```python
from build123d import *

# Parameters (mm, degrees)
SKETCH1_W           = 48
SKETCH1_H           = 300
SKETCH1_R           = 7
SKETCH1_R_2         = 2
BOSS_EXTRUDE1_DEPTH = 5
CHAMFER1_SIZE       = 3
CUT_EXTRUDE1_DEPTH  = 304.856874202


with BuildPart() as part:
    # Sketch1 → Boss-Extrude1 (new body)
    with BuildSketch(Plane.XY):
        with Locations((24, -150)):
            Rectangle(SKETCH1_W, SKETCH1_H)
        with Locations((24, -160)):
            Circle(SKETCH1_R, mode=Mode.SUBTRACT)
        with Locations((8, -144)):
            Circle(SKETCH1_R_2, mode=Mode.SUBTRACT)
        with Locations((16, -144)):
            Circle(SKETCH1_R_2, mode=Mode.SUBTRACT)
        with Locations((24, -144)):
            Circle(SKETCH1_R_2, mode=Mode.SUBTRACT)
        with Locations((32, -144)):
            Circle(SKETCH1_R_2, mode=Mode.SUBTRACT)
        with Locations((40, -144)):
            Circle(SKETCH1_R_2, mode=Mode.SUBTRACT)
        with Locations((16, -152)):
            Circle(SKETCH1_R_2, mode=Mode.SUBTRACT)
        with Locations((32, -152)):
            Circle(SKETCH1_R_2, mode=Mode.SUBTRACT)
        with Locations((40, -152)):
            Circle(SKETCH1_R_2, mode=Mode.SUBTRACT)
        with Locations((40, -160)):
            Circle(SKETCH1_R_2, mode=Mode.SUBTRACT)
        with Locations((16, -168)):
            Circle(SKETCH1_R_2, mode=Mode.SUBTRACT)
        with Locations((32, -168)):
            Circle(SKETCH1_R_2, mode=Mode.SUBTRACT)
        with Locations((40, -168)):
            Circle(SKETCH1_R_2, mode=Mode.SUBTRACT)
        with Locations((16, -176)):
            Circle(SKETCH1_R_2, mode=Mode.SUBTRACT)
        with Locations((24, -176)):
            Circle(SKETCH1_R_2, mode=Mode.SUBTRACT)
        with Locations((32, -176)):
            Circle(SKETCH1_R_2, mode=Mode.SUBTRACT)
        with Locations((40, -176)):
            Circle(SKETCH1_R_2, mode=Mode.SUBTRACT)
        with Locations((8, -152)):
            Circle(SKETCH1_R_2, mode=Mode.SUBTRACT)
        with Locations((8, -160)):
            Circle(SKETCH1_R_2, mode=Mode.SUBTRACT)
        with Locations((8, -168)):
            Circle(SKETCH1_R_2, mode=Mode.SUBTRACT)
        with Locations((8, -176)):
            Circle(SKETCH1_R_2, mode=Mode.SUBTRACT)
    extrude(amount=BOSS_EXTRUDE1_DEPTH)

    # Chamfer1
    chamfer1_edges = [part.edges().sort_by_distance(p)[0] for p in [
        (48, 0, 2.5),
        (0, 0, 2.5),
    ]]
    chamfer(chamfer1_edges, length=CHAMFER1_SIZE)

    # Sketch2 → Cut-Extrude1 (cut, through all)
    with BuildSketch(Plane.XY.offset(5)):
        with BuildLine():
            Line((14, -265), (14, -300))
            Line((14, -300), (34, -300))
            Line((34, -300), (34, -265))
            ThreePointArc((34, -265), (24, -255), (14, -265))
        make_face()
    extrude(amount=-CUT_EXTRUDE1_DEPTH, mode=Mode.SUBTRACT)


solid = part.part
```
Geometry check sheet. Reference: the model listing, model coordinates, mm. A direction names the side the tool comes from. Coordinates: 2 decimals unless noted, no trailing zeros.
Item 1: Sectioned sample at A-A, the plane z = 2.8. Count the separate pieces of the cut face and the enclosed holes in it, then the cut area to 3 significant figures.
Item 2: Thickness scan on line 1 (X direction, y = -176, z = 1.85); line 2 (X direction, y = -168, z = 2.5); line 3 (Y direction, x = 40, z = 2.4). Record the ranges inside material, lowest first.
Item 3: Access from +Z, -Z, +X, -X, +Y, -Y to the whole of each face (thin tool, end or side, straight path). Record for faces 4 (the face through (22.483, -166.834, 2.465)), 5 (the face through (34, -283, 3)).
Item 4: Release check for a two-part mould opening along X. For faces 1 (the face through (0, -154, 2)), 2 (the face through (24, -148, 0)), 3 (the face through (14, -282, 3)) record: released by +X, released by -X, zero draft, split by the parting line, or undercut.
Check result:
1. separate pieces: 1
1. enclosed holes: 21
1. area: 13,100 mm2
2. line 1: x = 0 to 6, 10 to 14, 18 to 22, 26 to 30, 34 to 38, 42 to 48
2. line 2: x = 0 to 6, 10 to 14, 18 to 30, 34 to 38, 42 to 48
2. line 3: y = -300 to -178, -174 to -170, -166 to -162, -158 to -154, -150 to -146, -142 to 0
3. face 4: +Z, -Z
3. face 5: +Z, -Z, -Y
4. face 1: released by -X
4. face 2: zero draft
4. face 3: undercut
